Geometry check sheet. Reference: the model listing, model coordinates, mm. Face numbers are marked on the shaded views. A direction names the side the tool comes from. Coordinates: 2 decimals unless noted, no trailing zeros. Loops run counter-clockwise (first coordinate to the right, second up) from the corner with the lowest first, then second, coordinate; pieces in that order, holes last.
from build123d import *

# Parameters (mm, degrees)
BASES_W                              = 19.4
BASES_H                              = 40.3
BASE_DEPTH                           = 8.6
SHAFTHOLES_R                         = 3
SHAFT_HOLE_DEPTH                     = 24.959810099
MOUNTINGTABS_W                       = 17.4
MOUNTINGTABS_H                       = 2.45
MOUNTING_TAB_DEPTH                   = 6.8
MOUNTING_HOLE_DEPTH                  = 30.295306791
BOTTOMALIGNHOLES_R                   = 0.7
BOTTOM_ALIGN_HOLE_DEPTH              = 0.5
TRIANGULAR_TAB_DEPTH                 = 0.9
MOUNTING_TAB_FEATURES_M_COPY_1_DEPTH = 30.295306791
BASE_START                           = 1.8
BASETOPBODYS_R                       = 3
BASE_TOP_BODY_DEPTH                  = 1.8
PART_CIRCLE_DEPTH                    = 1.8
TOP_START                            = 1.15
TOPBODYCYLINDER1_R                   = 6.4
TOPBODYCYLINDER1_R_2                 = 3
TOP_BODY_CYLINDER_1_DEPTH            = 1.15
TOB_START                            = 0.8
TOPBODYCYLINDER2_R                   = 5.6
TOPBODYCYLINDER2_R_2                 = 3
TOB_BODY_CYLINDER_2_DEPTH            = 0.8
TOPBODYLABELNEST_W                   = 17.8
TOPBODYLABELNEST_H                   = 12.5
TOPBODYLABELNEST_W_2                 = 15.6
TOPBODYLABELNEST_H_2                 = 10.3
TOP_BODY_LABEL_NEST_DEPTH            = 0.3
PART_CIRCLE_2_DEPTH                  = 0.3
BORDERCUTS_W                         = 19.4
BORDERCUTS_H                         = 40.3
BORDERCUTS_W_2                       = 18.8
BORDERCUTS_H_2                       = 39.7
BORDER_CUT_DEPTH                     = 0.5
MAIN_BODY_FEATURES_F_R               = 1
BORDER_CUT_F_R                       = 0.75


with BuildPart() as part:
    # BaseS → BASE (new body)
    with BuildSketch(Plane(origin=(0, 0, 0), x_dir=(1, 0, 0), z_dir=(0, 1, 0))):
        Rectangle(BASES_W, BASES_H)
    extrude(amount=BASE_DEPTH)

    # ShaftHoleS → SHAFT HOLE (cut, through all)
    with BuildSketch(Plane(origin=(0, 8.6, 0), x_dir=(1, 0, 0), z_dir=(0, 1, 0))):
        with Locations(Location((0, 10.15, 0), (0, 0, 270))):
            Circle(SHAFTHOLES_R)
    extrude(amount=-SHAFT_HOLE_DEPTH, mode=Mode.SUBTRACT)

    # MountingTabS → MOUNTING TAB (add)
    with BuildSketch(Plane.XY.offset(20.15)):
        with Locations((0, 1.225)):
            Rectangle(MOUNTINGTABS_W, MOUNTINGTABS_H)
    mounting_tab = extrude(amount=MOUNTING_TAB_DEPTH)

    # MountingHoleS → MOUNTING HOLE (cut, through all)
    with BuildSketch(Plane(origin=(0, 2.45, 0), x_dir=(1, 0, 0), z_dir=(0, 1, 0))):
        with BuildLine():
            Line((-6, -26.049193338), (-6, -26.95))
            Line((-6, -26.95), (-3.8, -26.95))
            Line((-3.8, -26.95), (-3.8, -26.049193338))
            ThreePointArc((-3.8, -26.049193338), (-4.9, -22.6), (-6, -26.049193338))
        make_face()
    mounting_hole = extrude(amount=-MOUNTING_HOLE_DEPTH, mode=Mode.SUBTRACT)

    # MH M: MOUNTING HOLE across plane
    add(mounting_hole.mirror(Plane(origin=(0, 0, 0), x_dir=(0, 0, 1), z_dir=(1, 0, 0))), mode=Mode.SUBTRACT)

    # BottomAlignHoleS → BOTTOM ALIGN HOLE (cut)
    with BuildSketch(Plane.XZ):
        with Locations(Location((0, 24.95, 0), (0, 0, 270))):
            Circle(BOTTOMALIGNHOLES_R)
    bottom_align_hole = extrude(amount=-BOTTOM_ALIGN_HOLE_DEPTH, mode=Mode.SUBTRACT)

    # TriangularTabS → TRIANGULAR TAB (add, symmetric)
    with BuildSketch(Plane(origin=(0, 0, 0), x_dir=(0, 0, -1), z_dir=(1, 0, 0))):
        Polygon((-20.15, 2.45), (-26.95, 2.45), (-20.15, 3.25), align=None)
    triangular_tab = extrude(amount=TRIANGULAR_TAB_DEPTH, both=True)

    # MOUNTING TAB FEATURES M: MOUNTING TAB, MOUNTING HOLE, BOTTOM ALIGN HOLE, TRIANGULAR TAB across plane
    add(mounting_tab.mirror(Plane.XY))
    add(mounting_hole.mirror(Plane.XY), mode=Mode.SUBTRACT)
    add(bottom_align_hole.mirror(Plane.XY), mode=Mode.SUBTRACT)
    add(triangular_tab.mirror(Plane.XY))

    # MOUNTING TAB FEATURES M copy 1 sketch → MOUNTING TAB FEATURES M copy 1 (cut, through all)
    with BuildSketch(Plane(origin=(0, 2.45, 0), x_dir=(-1, 0, 0), z_dir=(0, 1, 0))):
        with BuildLine():
            Line((-6, -26.049193338), (-6, -26.95))
            Line((-6, -26.95), (-3.8, -26.95))
            Line((-3.8, -26.95), (-3.8, -26.049193338))
            ThreePointArc((-3.8, -26.049193338), (-4.9, -22.6), (-6, -26.049193338))
        make_face()
    extrude(amount=-MOUNTING_TAB_FEATURES_M_COPY_1_DEPTH, mode=Mode.SUBTRACT)

    # BaseTopBodyS → BASE TOP BODY (add)
    with BuildSketch(Plane(origin=(0, 8.6, 0), x_dir=(1, 0, 0), z_dir=(0, 1, 0)).offset(BASE_START)):
        with BuildLine():
            Line((-8.9, -13.748610843), (8.9, -13.748610843))
            Line((8.9, -13.748610843), (8.9, 6.551389157))
            ThreePointArc((8.9, 6.551389157), (0, 19.75), (-8.9, 6.551389157))
            Line((-8.9, 6.551389157), (-8.9, -13.748610843))
        make_face()
        with Locations(Location((0, 10.15, 0), (0, 0, 270))):
            Circle(BASETOPBODYS_R, mode=Mode.SUBTRACT)
    extrude(amount=-BASE_TOP_BODY_DEPTH)

    # PartCircleS → PART CIRCLE (add)
    with BuildSketch(Plane(origin=(0, 8.6, 0), x_dir=(1, 0, 0), z_dir=(0, 1, 0))):
        with BuildLine():
            Line((-4.7, -13.748610843), (4.7, -13.748610843))
            ThreePointArc((4.7, -13.748610843), (0, -15.948610843), (-4.7, -13.748610843))
        make_face()
    extrude(amount=PART_CIRCLE_DEPTH)

    # TopBodyCylinder1 → TOP BODY CYLINDER 1 (add)
    with BuildSketch(Plane(origin=(0, 10.4, 0), x_dir=(1, 0, 0), z_dir=(0, 1, 0)).offset(TOP_START)):
        with Locations(Location((0, 10.15, 0), (0, 0, 270))):
            Circle(TOPBODYCYLINDER1_R)
        with Locations(Location((0, 10.15, 0), (0, 0, 270))):
            Circle(TOPBODYCYLINDER1_R_2, mode=Mode.SUBTRACT)
    extrude(amount=-TOP_BODY_CYLINDER_1_DEPTH)

    # TopBodyCylinder2 → TOB BODY CYLINDER 2 (add)
    with BuildSketch(Plane(origin=(0, 11.55, 0), x_dir=(1, 0, 0), z_dir=(0, 1, 0)).offset(TOB_START)):
        with Locations(Location((0, 10.15, 0), (0, 0, 270))):
            Circle(TOPBODYCYLINDER2_R)
        with Locations(Location((0, 10.15, 0), (0, 0, 270))):
            Circle(TOPBODYCYLINDER2_R_2, mode=Mode.SUBTRACT)
    extrude(amount=-TOB_BODY_CYLINDER_2_DEPTH)

    # TopBodyLabelNest → TOP BODY LABEL NEST (add)
    with BuildSketch(Plane(origin=(0, 10.4, 0), x_dir=(1, 0, 0), z_dir=(0, 1, 0))):
        with Locations((0, -7.498610843)):
            Rectangle(TOPBODYLABELNEST_W, TOPBODYLABELNEST_H)
        with Locations((0, -7.498610843)):
            Rectangle(TOPBODYLABELNEST_W_2, TOPBODYLABELNEST_H_2, mode=Mode.SUBTRACT)
    extrude(amount=TOP_BODY_LABEL_NEST_DEPTH)

    # PartCircle2S → PART CIRCLE 2 (add)
    with BuildSketch(Plane(origin=(0, 10.4, 0), x_dir=(1, 0, 0), z_dir=(0, 1, 0))):
        with BuildLine():
            Line((1.303840481, -2.348610843), (-1.303840481, -2.348610843))
            ThreePointArc((-1.303840481, -2.348610843), (0, 1.051389157), (1.303840481, -2.348610843))
        make_face()
    extrude(amount=PART_CIRCLE_2_DEPTH)

    # BorderCutS → BORDER CUT (cut)
    with BuildSketch(Plane(origin=(0, 8.6, 0), x_dir=(1, 0, 0), z_dir=(0, 1, 0))):
        Rectangle(BORDERCUTS_W, BORDERCUTS_H)
        Rectangle(BORDERCUTS_W_2, BORDERCUTS_H_2, mode=Mode.SUBTRACT)
    extrude(amount=-BORDER_CUT_DEPTH, mode=Mode.SUBTRACT)

    # MAIN BODY FEATURES F
    main_body_features_f_edges = [part.edges().sort_by_distance(p)[0] for p in [
        (8.7, 1.225, -26.95),
        (-8.7, 1.225, -26.95),
        (-9.7, 4.05, -20.15),
        (9.7, 4.05, -20.15),
        (-8.9, 9.65, 13.748610843),
        (8.9, 9.65, 13.748610843),
        (-9.7, 4.05, 20.15),
        (9.7, 4.05, 20.15),
        (8.7, 1.225, 26.95),
        (-8.7, 1.225, 26.95),
    ]]
    fillet(main_body_features_f_edges, radius=MAIN_BODY_FEATURES_F_R - 0.0001)  # a hair under: the kernel refuses the full size

    # BORDER CUT F
    border_cut_f_edges = [part.edges().sort_by_distance(p)[0] for p in [
        (9.4, 8.35, -19.85),
        (9.4, 8.35, 19.85),
        (-9.4, 8.35, 19.85),
        (-9.4, 8.35, -19.85),
    ]]
    fillet(border_cut_f_edges, radius=BORDER_CUT_F_R)


solid = part.part
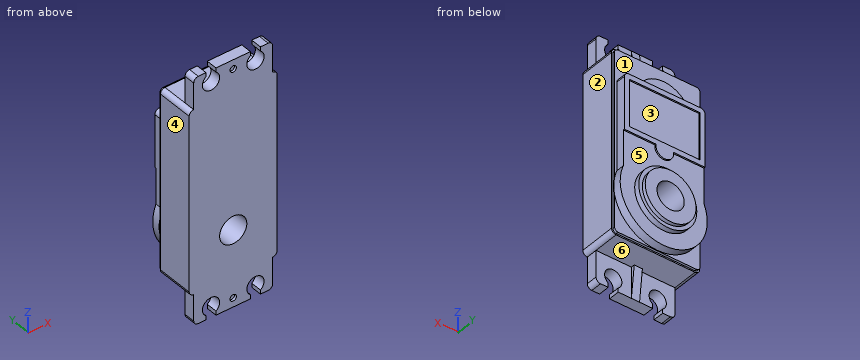
(1) Scan lines: L1, parallel to X at y = 1.8, z = 24.5; L2, parallel to X at y = 0.15, z = -24.95; L3, parallel to Z at x = -4.9, y = 1.8. Record each from-to range of solid material in increasing order.
Findings:
L1: x = -8.7 to -6.8, -3 to 3, 6.8 to 8.7
L2: x = -8.7 to -6.75, -3.05 to -0.7, 0.7 to 3.05, 6.75 to 8.7
L3: z = -22.6 to 22.6
(2) Sectioned sample at A-A on z = -10.15. Record the cut outline in (x, y).
Findings:
outline: (-9.7, 0) - (-3, 0) - (-3, 12.35) - (-5.6, 12.35) - (-5.6, 11.55) - (-6.4, 11.55) - (-6.4, 10.4) - (-9.6, 10.4) - (-9.6, 8.6) - (-9.4, 8.6) - (-9.4, 8.1) - (-9.7, 8.1) - close; (3, 0) - (9.7, 0) - (9.7, 8.1) - (9.4, 8.1) - (9.4, 8.6) - (9.6, 8.6) - (9.6, 10.4) - (6.4, 10.4) - (6.4, 11.55) - (5.6, 11.55) - (5.6, 12.35) - (3, 12.35) - close
(3) Access from +Z, -Z, +X, -X, +Y, -Y to the whole of each face (thin tool, end or side, straight path). Record for the marked faces 1, 2 and 3.
Findings:
face 1: +Z, +Y
face 2: +Z, -Z, +X, +Y, -Y
face 3: +Y
(4) Draft check along Z on the marked faces 4, 5 and 6. Enter one of: +Z half, -Z half, draft (parallel to the pull), parting line (faces both ways), or undercut.
Findings:
face 4: draft
face 5: undercut
face 6: -Z half
(5) Sectioned sample at C-C on z = 4. Record the cut outline in (x, y), and give its area (3 significant figures).
Findings:
outline: (-9.7, 0) - (9.7, 0) - (9.7, 8.1) - (9.4, 8.1) - (9.4, 8.6) - (8.9, 8.6) - (8.9, 10.7) - (7.8, 10.7) - (7.8, 10.4) - (-7.8, 10.4) - (-7.8, 10.7) - (-8.9, 10.7) - (-8.9, 8.6) - (-9.4, 8.6) - (-9.4, 8.1) - (-9.7, 8.1) - close
area: 199 mm2
(6) Gauge pin test, flat ends, axial feed: pin 1 Ø1 at (y, z) = (2, -26.5) entering from -X; pin 2 Ø3.5 at (x, z) = (-4.9, -24.5) entering from -Y; pin 3 Ø1 at (x, y) = (-7.5, 8) entering from -Z; pin 4 Ø2 at (y, z) = (10, -9.5) entering from +X. Record the tip position at first contact, or that the pin passes through.
Findings:
pin 1: stops at x = -8.7
pin 2: passes through
pin 3: stops at z = -20.15
pin 4: stops at x = 9.6
(7) Sectioned sample at D-D on z = 24.95. Record the cut outline in (x, y), and give its area (3 significant figures).
Findings:
outline: (-8.7, 0) - (-6.75, 0) - (-6.75, 2.45) - (-8.7, 2.45) - close; (-3.05, 0) - (-0.7, 0) - (-0.7, 0.5) - (0.7, 0.5) - (0.7, 0) - (3.05, 0) - (3.05, 2.45) - (0.9, 2.45) - (0.9, 2.69) - (-0.9, 2.69) - (-0.9, 2.45) - (-3.05, 2.45) - close; (6.75, 0) - (8.7, 0) - (8.7, 2.45) - (6.75, 2.45) - close
area: 24.3 mm2
(8) Sectioned sample at B-B on y = 5.75. Record the cut outline in (x, z).
Findings:
outline: (-9.7, -19.15) arc R1 ccw to (-8.7, -20.15) - (8.7, -20.15) arc R1 ccw to (9.7, -19.15) - (9.7, 19.15) arc R1 ccw to (8.7, 20.15) - (-8.7, 20.15) arc R1 ccw to (-9.7, 19.15) - close; hole circle Ø6 at (0, -10.15)
